Verification items for this drawing (mm, ordinates from the low corner). A direction names the side the tool comes from. Give positions to 0.01 mm unless a question says otherwise; leave off trailing zeros. Write each loop counter-clockwise with the first axis right and the second up, starting at its lowest first coordinate (ties: lowest second). Pieces come first, ordered by that corner, then holes. Notation, with made-up numbers: (31, 12) -> (76, 12) arc R18 cw to (76, 20) -> close; hole circle Ø5 at (-18.5, 22.25). An arc over 180 degrees is marked (long way). Answer as a JSON object with one key per item and string values.
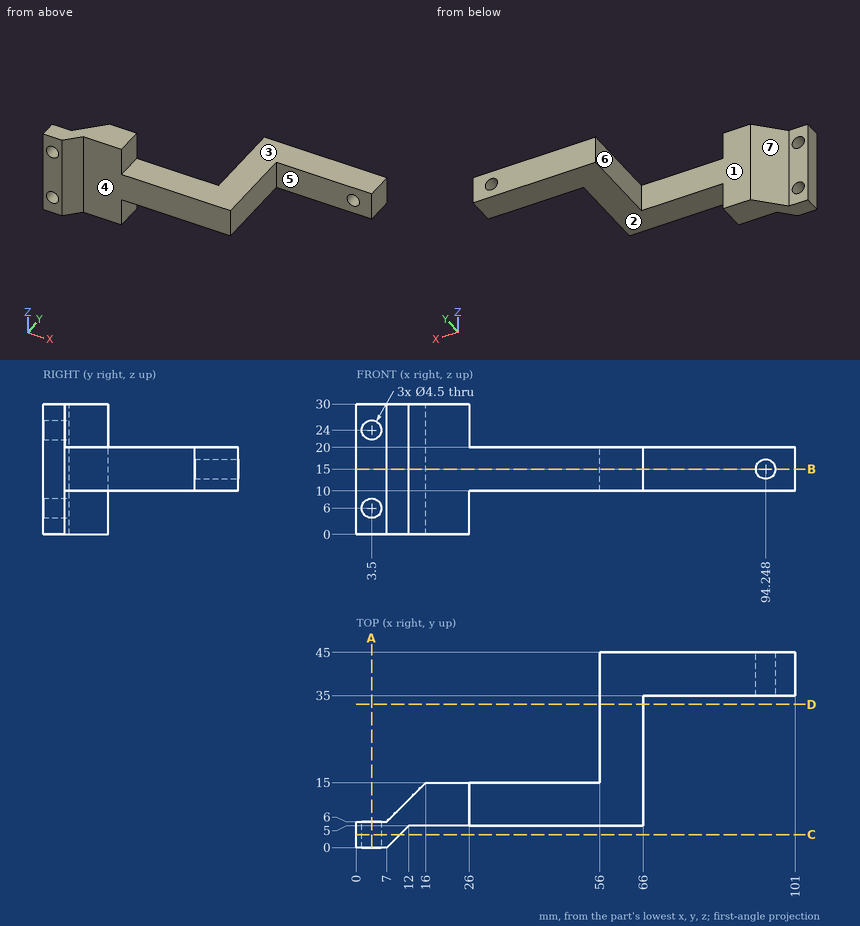
1. Sectioned sample at C-C, the plane y = 3. Enter the section's corners in (x, z).
Determined:
{"outline": "(0, 0) -> (10, 0) -> (10, 30) -> (0, 30) -> close; hole circle Ø4.5 at (3.5, 6); hole circle Ø4.5 at (3.5, 24)"}
2. Sectioned sample at A-A, the plane x = 3.5. Enter the section's corners in (y, z).
Determined:
{"outline": "(0, 0) -> (6, 0) -> (6, 3.75) -> (0, 3.75) -> close; (0, 8.25) -> (6, 8.25) -> (6, 21.75) -> (0, 21.75) -> close; (0, 26.25) -> (6, 26.25) -> (6, 30) -> (0, 30) -> close"}
3. Scan lines: L1, parallel to Z at x = 3.5, y = 3; L2, parallel to X at y = 39.5, z = 15; L3, parallel to Y at x = 28.5, z = 15.5. Record each from-to range of solid material in increasing order. Write a range as [from, to].
Determined:
{"L1": "[0, 3.75], [8.25, 21.75], [26.25, 30]", "L2": "[56, 92], [96.5, 101]", "L3": "[5, 15]"}
4. Sectioned sample at D-D, the plane y = 33. Enter the section's corners in (x, z), plus the area to 4 significant figures.
Determined:
{"outline": "(56, 10) -> (66, 10) -> (66, 20) -> (56, 20) -> close", "area": "100.0 mm^2"}
5. Mould release check, pull along Y, two halves, no side actions. Record for the marked faces 5, 6 and 7: released by +Y, released by -Y, zero draft, split by the parting line, or undercut.
Determined:
{"face 5": "released by -Y", "face 6": "zero draft", "face 7": "released by +Y"}
6. Sectioned sample at B-B, the plane z = 15. Enter the section's corners in (x, y).
Determined:
{"outline": "(0, 0) -> (7, 0) -> (12, 5) -> (66, 5) -> (66, 35) -> (92, 35) -> (92, 45) -> (56, 45) -> (56, 15) -> (16, 15) -> (7, 6) -> (0, 6) -> close; (96.5, 35) -> (101, 35) -> (101, 45) -> (96.5, 45) -> close"}
7. Go/stop test with flat-tipped pins: P1, Ø5, axis at x = 89.5, y = 33, coming from the +Z side; P2, Ø12, axis at y = 26, z = 18.5, coming from the -X side; P3, Ø11, axis at y = 8, z = 26.5, coming from the +X side; P4, Ø2.5, axis at x = 3.5, z = 6, coming from the +Y side. Record where each tip stops, or that it passes through.
Determined:
{"P1": "z = 20", "P2": "x = 56", "P3": "x = 26", "P4": "through"}
8. Access from +Z, -Z, +X, -X, +Y, -Y to the whole of each face (thin tool, end or side, straight path). Record for the marked faces 1, 2, 3 and 4.
Determined:
{"face 1": "+Z, -Z, -X, +Y", "face 2": "-Z, +X, +Y, -Y", "face 3": "+Z, +X, +Y, -Y", "face 4": "+Z, -Z, +X, -Y"}
